Can you work these out from the model? Positions are in its coordinate system, mm. Coordinates: 2 decimals unless noted, no trailing zeros. Order: outer loops, then holes, each group sorted by start corner. A loop starts at its lowest first (then second) coordinate and runs counter-clockwise, first axis right, second up. Notation, with made-up numbers: (-10.5, 37.25) - (2.5, 37.25) arc R19 ccw to (2.5, 49.25) - close; hole circle Ø7 at (-15.75, 22.5). An arc over 180 degrees is marked (long way). Return JSON: item names as keys, results as strings. Group by question number.
1) If I drill on line 1 along Z through (x, y) = (109.5, 1.6); line 2 along X through (y, z) = (0.3, -100); line 3 along Z through (x, y) = (238.5, 2.3), over which ranges is the centre line in solid material (lowest first)?
2) Imagine slicing it at B-B (x = 152). Write out the boundary of the cut face in (y, z).
3) Imagine slicing it at C-C (z = -8.5). Write out the boundary of the cut face in (x, y).
4) For pin 1 Ø4 at (x, z) = (304, -112.5) entering from -Y; pin 2 Ø1 at (x, y) = (216.5, 2) entering from -Z; pin 3 Ø1 at (x, y) = (197, 2.5) entering from -Z, each with a flat end and sliding along its axis, tell me the tip position at first contact or that it passes through.
5) Imagine slicing it at A-A (y = 2.4). Write out the boundary of the cut face in (x, z).
```python
from build123d import *

# Parameters (mm, degrees)
BOSS_EXTRUDE1_DEPTH = 3


with BuildPart() as part:
    # Sketch1 → Boss-Extrude1 (new body)
    with BuildSketch(Plane(origin=(0, 0, 0), x_dir=(1, 0, 0), z_dir=(0, 1, 0))):
        with BuildLine():
            Line((15, 0), (100, 0))
            Line((100, 0), (337.137947494, 34.147864439))
            ThreePointArc((337.137947494, 34.147864439), (346.33731036, 39.173042252), (350, 48.994722036))
            Line((350, 48.994722036), (350, 93.005277964))
            ThreePointArc((350, 93.005277964), (346.33731036, 102.826957748), (337.137947494, 107.852135561))
            Line((337.137947494, 107.852135561), (100, 142))
            Line((100, 142), (15, 142))
            ThreePointArc((15, 142), (4.393398282, 137.606601718), (0, 127))
            Line((0, 127), (0, 15))
            ThreePointArc((0, 15), (4.393398282, 4.393398282), (15, 0))
        make_face()
    extrude(amount=BOSS_EXTRUDE1_DEPTH)


solid = part.part
```
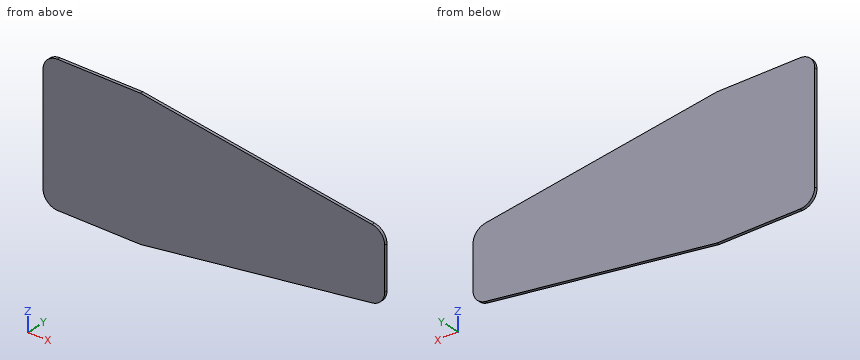
Calculated:
{
 "1": {"line 1": "-140.63 to -1.37", "line 2": "0 to 348.27", "line 3": "-122.06 to -19.94"},
 "2": {"outline": "(0, -134.51) - (3, -134.51) - (3, -7.49) - (0, -7.49) - close"},
 "3": {"outline": "(1.48, 0) - (159.03, 0) - (159.03, 3) - (1.48, 3) - close"},
 "4": {"pin 1": "y = 0", "pin 2": "z = -125.3", "pin 3": "z = -128.1"},
 "5": {"outline": "(0, -127) arc R15 ccw to (15, -142) - (100, -142) - (337.14, -107.85) arc R15 ccw to (350, -93.01) - (350, -48.99) arc R15 ccw to (337.14, -34.15) - (100, 0) - (15, 0) arc R15 ccw to (0, -15) - close"}
}
